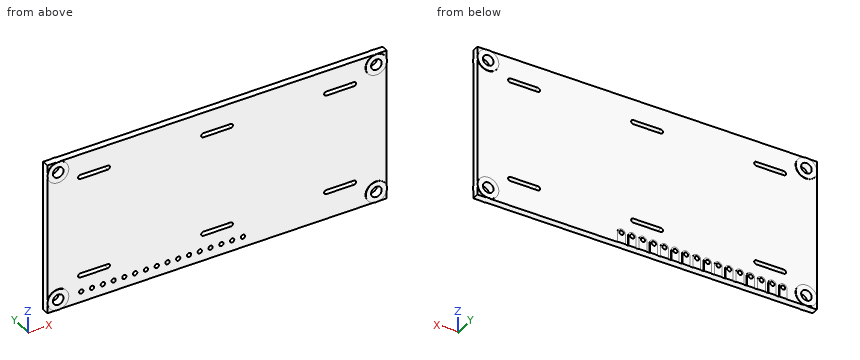
from build123d import *

# Parameters (mm, degrees)
SKETCH1_W           = 80
SKETCH1_H           = 36
SKETCH1_R           = 1.25
SKETCH1_R_2         = 0.5
BOSS_EXTRUDE1_DEPTH = 1.6
SKETCH2_R           = 0.5
BOSS_EXTRUDE2_DEPTH = 0.1
LPATTERN1_COUNT     = 16
LPATTERN1_PITCH     = 2.54
SKETCH3_R           = 2.5
SKETCH3_R_2         = 1.25
BOSS_EXTRUDE3_DEPTH = 0.1
SKETCH4_R           = 2.5
SKETCH4_R_2         = 1.25
BOSS_EXTRUDE4_DEPTH = 0.1


with BuildPart() as part:
    # Sketch1 → Boss-Extrude1 (new body)
    with BuildSketch(Plane(origin=(0, 0, 0), x_dir=(1, 0, 0), z_dir=(0, 1, 0))):
        Rectangle(SKETCH1_W, SKETCH1_H)
        with Locations((-37.5, 15.5)):
            Circle(SKETCH1_R, mode=Mode.SUBTRACT)
        with Locations((-37.5, -15.5)):
            Circle(SKETCH1_R, mode=Mode.SUBTRACT)
        with Locations((37.5, 15.5)):
            Circle(SKETCH1_R, mode=Mode.SUBTRACT)
        with Locations((37.5, -15.5)):
            Circle(SKETCH1_R, mode=Mode.SUBTRACT)
        with Locations((-32, 15.5)):
            Circle(SKETCH1_R_2, mode=Mode.SUBTRACT)
        with Locations((-29.46, 15.5)):
            Circle(SKETCH1_R_2, mode=Mode.SUBTRACT)
        with Locations((-26.92, 15.5)):
            Circle(SKETCH1_R_2, mode=Mode.SUBTRACT)
        with Locations((-24.38, 15.5)):
            Circle(SKETCH1_R_2, mode=Mode.SUBTRACT)
        with Locations((-21.84, 15.5)):
            Circle(SKETCH1_R_2, mode=Mode.SUBTRACT)
        with Locations((-19.3, 15.5)):
            Circle(SKETCH1_R_2, mode=Mode.SUBTRACT)
        with Locations((-16.76, 15.5)):
            Circle(SKETCH1_R_2, mode=Mode.SUBTRACT)
        with Locations((-14.22, 15.5)):
            Circle(SKETCH1_R_2, mode=Mode.SUBTRACT)
        with Locations((-11.68, 15.5)):
            Circle(SKETCH1_R_2, mode=Mode.SUBTRACT)
        with Locations((-9.14, 15.5)):
            Circle(SKETCH1_R_2, mode=Mode.SUBTRACT)
        with Locations((-6.6, 15.5)):
            Circle(SKETCH1_R_2, mode=Mode.SUBTRACT)
        with Locations((-4.06, 15.5)):
            Circle(SKETCH1_R_2, mode=Mode.SUBTRACT)
        with Locations((-1.52, 15.5)):
            Circle(SKETCH1_R_2, mode=Mode.SUBTRACT)
        with Locations((1.02, 15.5)):
            Circle(SKETCH1_R_2, mode=Mode.SUBTRACT)
        with Locations((3.56, 15.5)):
            Circle(SKETCH1_R_2, mode=Mode.SUBTRACT)
        with Locations((6.1, 15.5)):
            Circle(SKETCH1_R_2, mode=Mode.SUBTRACT)
        with BuildLine():
            Line((-3.25, -12), (3.25, -12))
            ThreePointArc((3.25, -12), (3.75, -12.5), (3.25, -13))
            Line((3.25, -13), (-3.25, -13))
            ThreePointArc((-3.25, -13), (-3.75, -12.5), (-3.25, -12))
        make_face(mode=Mode.SUBTRACT)
        with BuildLine():
            Line((25.75, -12), (32.25, -12))
            ThreePointArc((32.25, -12), (32.75, -12.5), (32.25, -13))
            Line((32.25, -13), (25.75, -13))
            ThreePointArc((25.75, -13), (25.25, -12.5), (25.75, -12))
        make_face(mode=Mode.SUBTRACT)
        with BuildLine():
            Line((25.75, 12), (32.25, 12))
            ThreePointArc((32.25, 12), (32.75, 11.5), (32.25, 11))
            Line((32.25, 11), (25.75, 11))
            ThreePointArc((25.75, 11), (25.25, 11.5), (25.75, 12))
        make_face(mode=Mode.SUBTRACT)
        with BuildLine():
            Line((-3.25, 12), (3.25, 12))
            ThreePointArc((3.25, 12), (3.75, 11.5), (3.25, 11))
            Line((3.25, 11), (-3.25, 11))
            ThreePointArc((-3.25, 11), (-3.75, 11.5), (-3.25, 12))
        make_face(mode=Mode.SUBTRACT)
        with BuildLine():
            Line((-32.25, -12), (-25.75, -12))
            ThreePointArc((-25.75, -12), (-25.25, -12.5), (-25.75, -13))
            Line((-25.75, -13), (-32.25, -13))
            ThreePointArc((-32.25, -13), (-32.75, -12.5), (-32.25, -12))
        make_face(mode=Mode.SUBTRACT)
        with BuildLine():
            Line((-32.25, 12), (-25.75, 12))
            ThreePointArc((-25.75, 12), (-25.25, 11.5), (-25.75, 11))
            Line((-25.75, 11), (-32.25, 11))
            ThreePointArc((-32.25, 11), (-32.75, 11.5), (-32.25, 12))
        make_face(mode=Mode.SUBTRACT)
    extrude(amount=-BOSS_EXTRUDE1_DEPTH)

    # Sketch2 → Boss-Extrude2 (add)
    with BuildSketch(Plane(origin=(0, 0, 0), x_dir=(1, 0, 0), z_dir=(0, 1, 0))):
        with BuildLine():
            Line((-32.9, 15.5), (-32.9, 18))
            Line((-32.9, 18), (-31.1, 18))
            Line((-31.1, 18), (-31.1, 15.5))
            ThreePointArc((-31.1, 15.5), (-32, 14.6), (-32.9, 15.5))
        make_face()
        with Locations((-32, 15.5)):
            Circle(SKETCH2_R, mode=Mode.SUBTRACT)
    boss_extrude2 = extrude(amount=BOSS_EXTRUDE2_DEPTH)

    # LPattern1: Boss-Extrude2 ×16
    with Locations(*[(i * LPATTERN1_PITCH, 0, 0) for i in range(1, LPATTERN1_COUNT)]):
        add(boss_extrude2)

    # Sketch3 → Boss-Extrude3 (add)
    with BuildSketch(Plane(origin=(0, 0, 0), x_dir=(1, 0, 0), z_dir=(0, 1, 0))):
        with Locations((-37.5, 15.5)):
            Circle(SKETCH3_R)
        with Locations((-37.5, 15.5)):
            Circle(SKETCH3_R_2, mode=Mode.SUBTRACT)
        with Locations((-37.5, -15.5)):
            Circle(SKETCH3_R)
        with Locations((-37.5, -15.5)):
            Circle(SKETCH3_R_2, mode=Mode.SUBTRACT)
        with Locations((37.5, -15.5)):
            Circle(SKETCH3_R)
        with Locations((37.5, -15.5)):
            Circle(SKETCH3_R_2, mode=Mode.SUBTRACT)
        with Locations((37.5, 15.5)):
            Circle(SKETCH3_R)
        with Locations((37.5, 15.5)):
            Circle(SKETCH3_R_2, mode=Mode.SUBTRACT)
    extrude(amount=BOSS_EXTRUDE3_DEPTH)

    # Sketch4 → Boss-Extrude4 (add)
    with BuildSketch(Plane.XZ.offset(1.6)):
        with Locations((37.5, -15.5)):
            Circle(SKETCH4_R)
        with Locations((37.5, -15.5)):
            Circle(SKETCH4_R_2, mode=Mode.SUBTRACT)
        with Locations((37.5, 15.5)):
            Circle(SKETCH4_R)
        with Locations((37.5, 15.5)):
            Circle(SKETCH4_R_2, mode=Mode.SUBTRACT)
        with Locations((-37.5, 15.5)):
            Circle(SKETCH4_R)
        with Locations((-37.5, 15.5)):
            Circle(SKETCH4_R_2, mode=Mode.SUBTRACT)
        with Locations((-37.5, -15.5)):
            Circle(SKETCH4_R)
        with Locations((-37.5, -15.5)):
            Circle(SKETCH4_R_2, mode=Mode.SUBTRACT)
    extrude(amount=BOSS_EXTRUDE4_DEPTH)


solid = part.part
Source: CAD feature listing. Evaluate the final solid. Frame: model axes, mm. Give positions to 0.01 mm unless a question says otherwise; leave off trailing zeros. Order: outer loops, then holes, each group sorted by start corner. A loop starts at its lowest first (then second) coordinate and runs counter-clockwise, first axis right, second up. Notation, with made-up numbers: (9.25, 34.5) -> (41.25, 34.5) arc R18 cw to (41.25, 40.5) -> close; hole circle Ø9 at (53, -7.75). An arc over 180 degrees is marked (long way). Use a Markdown table: item, result.
1) Ray query, line 1 along Z through (x, y) = (26.5, -0.3); line 2 along Z through (x, y) = (-21.84, 0.05); line 3 along Z through (x, y) = (-29.46, -0.4). Return the intervals inside material, ascending. Write a range as [from, to].
Answer list:
| item | result |
|---|---|
| line 1 | [-18, -12], [-11, 12], [13, 18] |
| line 2 | [-18, -16], [-15, -14.6] |
| line 3 | [-18, -16], [-15, -12], [-11, 12], [13, 18] |
2) Section query A-A, the plane x = 28. Return the cut outline in (y, z), then the cut area to 3 significant figures.
Answer list:
| item | result |
|---|---|
| outline | (-1.6, -18) -> (0, -18) -> (0, -12) -> (-1.6, -12) -> close; (-1.6, -11) -> (0, -11) -> (0, 12) -> (-1.6, 12) -> close; (-1.6, 13) -> (0, 13) -> (0, 18) -> (-1.6, 18) -> close |
| area | 54.4 mm² |
3) Section query C-C, the plane z = 3.5. Return the cut outline in (x, y), then the cut area to 3 significant figures.
Answer list:
| item | result |
|---|---|
| outline | (-40, -1.6) -> (40, -1.6) -> (40, 0) -> (-40, 0) -> close |
| area | 128 mm² |
4) Section query B-B, the plane y = -1.25. Count the separate pieces of the cut face and the enclosed holes in it, then the cut area to 3 significant figures.
Answer list:
| item | result |
|---|---|
| separate pieces | 1 |
| enclosed holes | 26 |
| area | 2,800 mm² |
5) Contact query for flat-ended pins moving along their axis: P1, Ø11, axis at x = 4.5, z = -8, coming from the +Y side; P2, Ø1.5, axis at x = 19.5, z = 9.5, coming from the -Y side. Output: stop coordinate, or through.
Answer list:
| item | result |
|---|---|
| P1 | y = 0 |
| P2 | y = -1.6 |
